Source: CAD feature listing. Evaluate the final solid. Frame: model axes, mm. Face numbers are marked on the shaded views. Give positions to 0.01 mm unless a question says otherwise; leave off trailing zeros. Order: outer loops, then holes, each group sorted by start corner. A loop starts at its lowest first (then second) coordinate and runs counter-clockwise, first axis right, second up. Notation, with made-up numbers: (44, -10.75) -> (99, -10.75) arc R11 ccw to (99, 0.25) -> close; hole circle Ø2 at (-10, -5.5). An arc over 180 degrees is marked (long way). Answer in a Markdown table with one row per item.
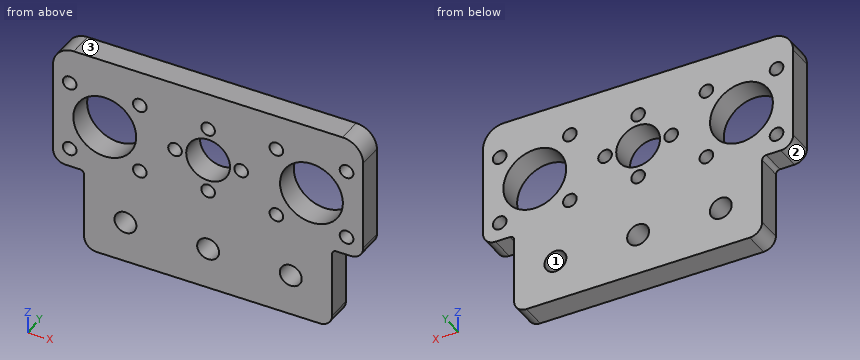
```python
from build123d import *

# Parameters (mm, degrees)
SKETCH_1_R      = 1.65
SKETCH_1_R_2    = 7.6
SKETCH_1_R_3    = 5.3
SKETCH_1_R_4    = 2.65
EXTRUDE_1_DEPTH = 6
FILLET_1_R      = 3
FILLET_2_R      = 1


with BuildPart() as part:
    # 草图1 → 凸台-拉伸1 (new body)
    with BuildSketch(Plane(origin=(0, 0, 0), x_dir=(1, 0, 0), z_dir=(0, 1, 0))):
        with BuildLine():
            Line((-30, 13), (-37.5, 13))
            Line((-37.5, 13), (-37.5, -12))
            ThreePointArc((-37.5, -12), (-36.035533906, -15.535533906), (-32.5, -17))
            Line((-32.5, -17), (32.5, -17))
            ThreePointArc((32.5, -17), (36.035533906, -15.535533906), (37.5, -12))
            Line((37.5, -12), (37.5, 13))
            Line((37.5, 13), (30, 13))
            Line((30, 13), (30, 33))
            Line((30, 33), (-30, 33))
            Line((-30, 33), (-30, 13))
        make_face()
        with Locations(Location((-33.485281374, -8.485281374, 0), (0, 0, 270))):
            Circle(SKETCH_1_R, mode=Mode.SUBTRACT)
        with Locations(Location((-16.514718626, -8.485281374, 0), (0, 0, 270))):
            Circle(SKETCH_1_R, mode=Mode.SUBTRACT)
        with Locations(Location((0, -8, 0), (0, 0, 270))):
            Circle(SKETCH_1_R, mode=Mode.SUBTRACT)
        with Locations(Location((-25, 0, 0), (0, 0, 270))):
            Circle(SKETCH_1_R_2, mode=Mode.SUBTRACT)
        with Locations(Location((-8, 0, 0), (0, 0, 270))):
            Circle(SKETCH_1_R, mode=Mode.SUBTRACT)
        with Locations(Location((0, 0, 0), (0, 0, 270))):
            Circle(SKETCH_1_R_3, mode=Mode.SUBTRACT)
        with Locations(Location((0, 8, 0), (0, 0, 270))):
            Circle(SKETCH_1_R, mode=Mode.SUBTRACT)
        with Locations(Location((16.514718626, -8.485281374, 0), (0, 0, 270))):
            Circle(SKETCH_1_R, mode=Mode.SUBTRACT)
        with Locations(Location((33.485281374, -8.485281374, 0), (0, 0, 270))):
            Circle(SKETCH_1_R, mode=Mode.SUBTRACT)
        with Locations(Location((8, 0, 0), (0, 0, 270))):
            Circle(SKETCH_1_R, mode=Mode.SUBTRACT)
        with Locations(Location((25, 0, 0), (0, 0, 270))):
            Circle(SKETCH_1_R_2, mode=Mode.SUBTRACT)
        with Locations(Location((-33.485281374, 8.485281374, 0), (0, 0, 270))):
            Circle(SKETCH_1_R, mode=Mode.SUBTRACT)
        with Locations(Location((-16.514718626, 8.485281374, 0), (0, 0, 270))):
            Circle(SKETCH_1_R, mode=Mode.SUBTRACT)
        with Locations(Location((-20, 23, 0), (0, 0, 270))):
            Circle(SKETCH_1_R_4, mode=Mode.SUBTRACT)
        with Locations(Location((0, 23, 0), (0, 0, 270))):
            Circle(SKETCH_1_R_4, mode=Mode.SUBTRACT)
        with Locations(Location((16.514718626, 8.485281374, 0), (0, 0, 270))):
            Circle(SKETCH_1_R, mode=Mode.SUBTRACT)
        with Locations(Location((33.485281374, 8.485281374, 0), (0, 0, 270))):
            Circle(SKETCH_1_R, mode=Mode.SUBTRACT)
        with Locations(Location((20, 23, 0), (0, 0, 270))):
            Circle(SKETCH_1_R_4, mode=Mode.SUBTRACT)
    extrude(amount=EXTRUDE_1_DEPTH)

    # 圆角1
    fillet_1_edges = [part.edges().sort_by_distance(p)[0] for p in [
        (-37.5, 3, -13),
        (-30, 3, -33),
        (30, 3, -33),
        (37.5, 3, -13),
    ]]
    fillet(fillet_1_edges, radius=FILLET_1_R)

    # 圆角2
    fillet_2_edges = [part.edges().sort_by_distance(p)[0] for p in [
        (-30, 3, -13),
        (30, 3, -13),
    ]]
    fillet(fillet_2_edges, radius=FILLET_2_R)


solid = part.part
```
(1) First-contact query: pin 1 Ø1.8 at (x, y) = (-33, 3.5) entering from -Z. Flat tip, straight axial feed; report the tip coordinate or a pass-through.
A:
| item | result |
|---|---|
| pin 1 | stops at z = -13 |
(2) Section query D-D (y = 3.7). Give the number of separate pieces and of enclosed holes in the cut face, plus the area to 3 significant figures.
A:
| item | result |
|---|---|
| separate pieces | 1 |
| enclosed holes | 18 |
| area | 2,810 mm^2 |
(3) Ray query, probe 1 along X at (y, z) = (2.55, 0); probe 2 along X at (y, z) = (4.35, -23); probe 3 along X at (y, z) = (0.55, -10). Return the intervals inside material, ascending.
A:
| item | result |
|---|---|
| probe 1 | x = -37.5 to -32.6, -17.4 to -9.65, -6.35 to -5.3, 5.3 to 6.35, 9.65 to 17.4, 32.6 to 37.5 |
| probe 2 | x = -30 to -22.65, -17.35 to -2.65, 2.65 to 17.35, 22.65 to 30 |
| probe 3 | x = -37.5 to -34.14, -32.83 to -17.17, -15.86 to 15.86, 17.17 to 32.83, 34.14 to 37.5 |
(4) Pull-direction query (X, two-part tool) for the marked faces 1, 2 and 3; classes: +X half, -X half, draft (parallel to the pull), parting line (faces both ways), or undercut.
A:
| item | result |
|---|---|
| face 1 | undercut |
| face 2 | -X half |
| face 3 | draft |
(5) Section query C-C (x = 0). Return the cut outline in (y, z).
A:
| item | result |
|---|---|
| outline | (0, -33) -> (6, -33) -> (6, -25.65) -> (0, -25.65) -> close; (0, -20.35) -> (6, -20.35) -> (6, -9.65) -> (0, -9.65) -> close; (0, -6.35) -> (6, -6.35) -> (6, -5.3) -> (0, -5.3) -> close; (0, 5.3) -> (6, 5.3) -> (6, 6.35) -> (0, 6.35) -> close; (0, 9.65) -> (6, 9.65) -> (6, 17) -> (0, 17) -> close |
(6) Section query B-B (z = -23). Return the cut outline in (x, y), plus the area to 3 significant figures.
A:
| item | result |
|---|---|
| outline | (-30, 0) -> (-22.65, 0) -> (-22.65, 6) -> (-30, 6) -> close; (-17.35, 0) -> (-2.65, 0) -> (-2.65, 6) -> (-17.35, 6) -> close; (2.65, 0) -> (17.35, 0) -> (17.35, 6) -> (2.65, 6) -> close; (22.65, 0) -> (30, 0) -> (30, 6) -> (22.65, 6) -> close |
| area | 265 mm^2 |
(7) Section query A-A (x = 25). Return the cut outline in (y, z).
A:
| item | result |
|---|---|
| outline | (0, -33) -> (6, -33) -> (6, -7.6) -> (0, -7.6) -> close; (0, 7.6) -> (6, 7.6) -> (6, 17) -> (0, 17) -> close |
